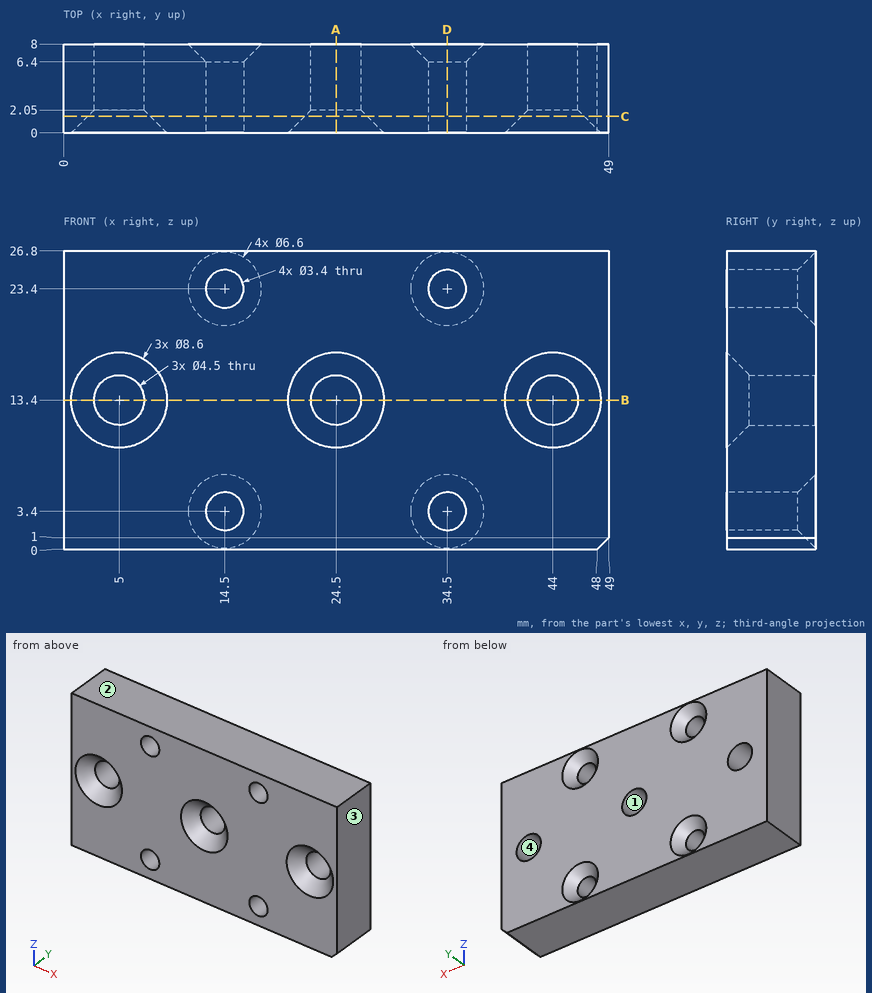
Answer from the drawing. Dimensions are ordinates in mm from the lowest x, y and z of the part. Round coordinates to 2 decimals unless told otherwise and drop trailing zeros. Loops run counter-clockwise (first coordinate to the right, second up) from the corner with the lowest first, then second, coordinate; pieces in that order, holes last.
(1) Each of these flat-tipped pins is pushed along its axis until it touches: P1, Ø5, axis at x = 24.5, z = 13.4, coming from the -Y side; P2, Ø2, axis at x = 34.5, z = 23.4, coming from the +Y side. Where does it stop, or does it pass through?
Computed values:
P1: stops at y = 1.8
P2: passes through
(2) The part is cut by section C-C, the plane y = 1.5. Give the vertices of the cut face in (x, z).
Computed values:
outline: (0, 0) - (48, 0) - (49, 1) - (49, 26.8) - (0, 26.8) - close; hole circle Ø5.6 at (5, 13.4); hole circle Ø3.4 at (14.5, 3.4); hole circle Ø3.4 at (14.5, 23.4); hole circle Ø5.6 at (24.5, 13.4); hole circle Ø3.4 at (34.5, 3.4); hole circle Ø3.4 at (34.5, 23.4); hole circle Ø5.6 at (44, 13.4)
(3) The mould has two halves that part along X. Classify the marked faces 1, 2, 3 and 4: pulls with the +X half, pulls with the -X half, needs draft (parallel to the pull), parting line crosses it, or undercut.
Computed values:
face 1: undercut
face 2: needs draft
face 3: pulls with the +X half
face 4: undercut
(4) The part is cut by section B-B, the plane z = 13.4. Give the vertices of the cut face in (x, y).
Computed values:
outline: (0, 0) - (0.7, 0) - (2.75, 2.05) - (2.75, 8) - (0, 8) - close; (7.25, 2.05) - (9.3, 0) - (20.2, 0) - (22.25, 2.05) - (22.25, 8) - (7.25, 8) - close; (26.75, 2.05) - (28.8, 0) - (39.7, 0) - (41.75, 2.05) - (41.75, 8) - (26.75, 8) - close; (46.25, 2.05) - (48.3, 0) - (49, 0) - (49, 8) - (46.25, 8) - close
(5) The part is cut by section A-A, the plane x = 24.5. Give the vertices of the cut face in (y, z).
Computed values:
outline: (0, 0) - (8, 0) - (8, 11.15) - (2.05, 11.15) - (0, 9.1) - close; (0, 17.7) - (2.05, 15.65) - (8, 15.65) - (8, 26.8) - (0, 26.8) - close
(6) Find the intervals of material crossed by L1, parallel to X at y = 3, z = 23.4; L2, parallel to Z at x = 34.5, y = 2.75; L3, parallel to X at y = 5.6, z = 13.4, in increasing order.
Computed values:
L1: x = 0 to 12.8, 16.2 to 32.8, 36.2 to 49
L2: z = 0 to 1.7, 5.1 to 21.7, 25.1 to 26.8
L3: x = 0 to 2.75, 7.25 to 22.25, 26.75 to 41.75, 46.25 to 49
(7) The part is cut by section D-D, the plane x = 34.5. Give the vertices of the cut face in (y, z).
Computed values:
outline: (0, 0) - (8, 0) - (8, 0.1) - (6.4, 1.7) - (0, 1.7) - close; (0, 5.1) - (6.4, 5.1) - (8, 6.7) - (8, 20.1) - (6.4, 21.7) - (0, 21.7) - close; (0, 25.1) - (6.4, 25.1) - (8, 26.7) - (8, 26.8) - (0, 26.8) - close
